Geometry check sheet. Reference: drawing and pictorial views, mm from the part's lowest x, y, z. Give positions to 0.01 mm unless a question says otherwise; leave off trailing zeros. Order: outer loops, then holes, each group sorted by start corner. A loop starts at its lowest first (then second) coordinate and runs counter-clockwise, first axis right, second up. Notation, with made-up numbers: M -36,44.25 L 12,44.25 A12 cw 12,49.25 Z; hole C -39,33.5 d1. An arc over 180 degrees is marked long. Answer as a JSON object with one key per item and string values. Group by question number.
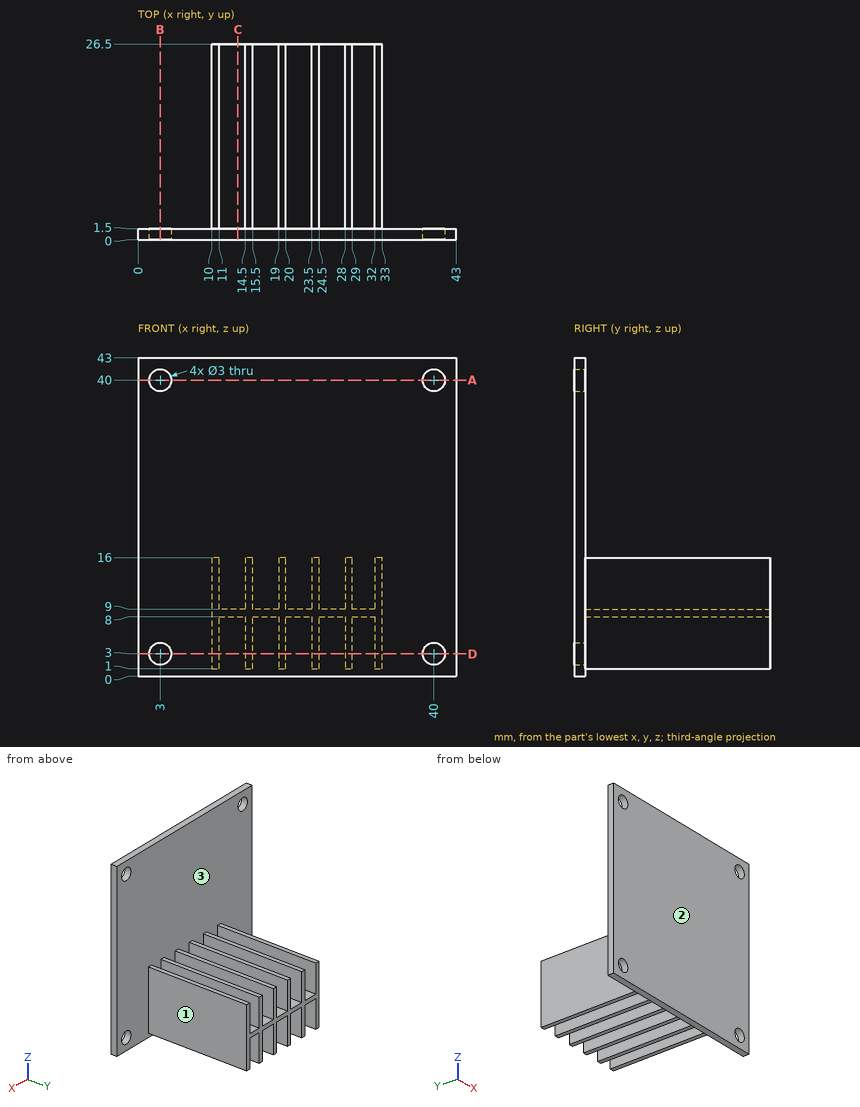
1. Cross-section at D-D (z = 3). State how many separate pieces and enclosed holes the cut face has, and give its area (4 significant figures).
2. Release check for a two-part mould opening along X. For the marked faces 1, 2 and 3 record: released by +X, released by -X, zero draft, split by the parting line, or undercut.
3. Cross-section at A-A (z = 40). Record the cut outline in (x, y).
4. Depth check by flat-ended pin: pin 1 (0.8 mm diameter, centred on x = 24, y = 9, fed in from +Z); pin 2 (10 mm diameter, centred on y = 11.5, z = 13.5, fed in from +X); pin 3 (0.8 mm diameter, centred on x = 28.5, y = 15, fed in from -Z); pin 4 (12 mm diameter, centred on x = 12, z = 13.5, fed in from +Y). Enter the tip coordinate at first touch or a pass-through.
5. Thickness scan on line 1 along Z through (x, y) = (40, 0.4); line 2 along X through (y, z) = (14, 9.5). Record the ranges inside material, lowest first. Write a range as [from, to].
6. Cross-section at C-C (x = 13.5). Record the cut outline in (y, z), and give its area (3 significant figures).
7. Cross-section at B-B (x = 3). Record the cut outline in (y, z), and give its area (3 significant figures).
Report:
{
 "1": {"separate pieces": "3", "enclosed holes": "0", "area": "205.5 mm2"},
 "2": {"face 1": "released by +X", "face 2": "zero draft", "face 3": "undercut"},
 "3": {"outline": "M 0,0 L 1.5,0 L 1.5,1.5 L 0,1.5 Z; M 4.5,0 L 38.5,0 L 38.5,1.5 L 4.5,1.5 Z; M 41.5,0 L 43,0 L 43,1.5 L 41.5,1.5 Z"},
 "4": {"pin 1": "stops at z = 16", "pin 2": "stops at x = 33", "pin 3": "stops at z = 1", "pin 4": "stops at y = 26.5"},
 "5": {"line 1": "z = [0, 1.5], [4.5, 38.5], [41.5, 43]", "line 2": "x = [10, 11], [14.5, 15.5], [19, 20], [23.5, 24.5], [28, 29], [32, 33]"},
 "6": {"outline": "M 0,0 L 1.5,0 L 1.5,8 L 26.5,8 L 26.5,9 L 1.5,9 L 1.5,43 L 0,43 Z", "area": "89.5 mm2"},
 "7": {"outline": "M 0,0 L 1.5,0 L 1.5,1.5 L 0,1.5 Z; M 0,4.5 L 1.5,4.5 L 1.5,38.5 L 0,38.5 Z; M 0,41.5 L 1.5,41.5 L 1.5,43 L 0,43 Z", "area": "55.5 mm2"}
}
